Geometry: final body of the model. Coordinates: model frame, mm. Face numbers are marked on the shaded views. Round coordinates to 2 decimals unless told otherwise and drop trailing zeros. Write each loop counter-clockwise with the first axis right and the second up, starting at its lowest first coordinate (ties: lowest second). Pieces come first, ordered by that corner, then holes. Notation, with made-up numbers: M 59,62 L 81,62 A12 ccw 81,68 Z; hole C 7.25,77.5 d5. An arc over 180 degrees is marked long. Use one line per item in the form item = value. Start each with the question number.
Item 1: Section query A-A (z = 0). Return loops of the section in (x, y), and give its area (3 significant figures).
Item 2: Pull-direction query (Z, two-part tool) for the marked faces 1, 2 and 3; classes: pulls with the +Z half, pulls with the -Z half, needs draft (parallel to the pull), parting line crosses it, or undercut.
Item 3: Pin query (flat end, axial travel): pin 1 Ø3 at (x, y) = (-11.5, -2.5) entering from +Z; pin 2 Ø2 at (x, y) = (-11.5, -4.5) entering from -Z; pin 3 Ø2 at (x, y) = (-9, -5) entering from +Z; pin 4 Ø5 at (x, y) = (-3, -2.5) entering from +Z (3 decimals). Return the tip coordinate at first contact, or that it passes through.
Item 4: Ray query, probe 1 along Z at (x, y) = (-15, -9.25); probe 2 along Z at (x, y) = (-8.75, -12.25); probe 3 along X at (y, z) = (-17.5, 2). Return the intervals inside material, ascending.
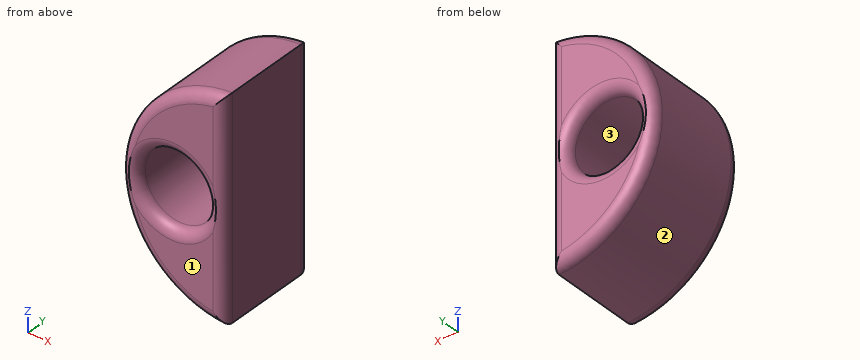
from build123d import *

# Parameters (mm, degrees)
F1_DEPTH    = 20
F2_R        = 6.5
F3_DEPTH    = 20
F4_T1_DEPTH = 49.9499687109
F4_T4_ANGLE = 202.9591024792
F4_T6_ANGLE = 202.9591024792


# Not quite as in the source:
# - a fillet or chamfer that OpenCascade refuses, or shapes differently, is made with other operations: its cross-section is extruded or revolved along the edge and cut away or added


with BuildPart() as f1:
    # F0 (on Front) → F1 (new body)
    with BuildSketch(Plane.XZ):
        with BuildLine():
            Line((-1, 0), (-1, 19.9749843554))
            ThreePointArc((-1, 19.9749843554), (-20, 0), (-1, -19.9749843554))
            Line((-1, -19.9749843554), (-1, 0))
        make_face()
    extrude(amount=F1_DEPTH)

    # F2 (on face) → F3 (cut)
    with BuildSketch(Plane.XZ.offset(20)):
        with Locations((-10.5, 0)):
            Circle(F2_R)
    extrude(amount=-F3_DEPTH, mode=Mode.SUBTRACT)

    # F4: fillet of radius 2 on 6 edges, made by hand

    # F4_s2 → F4_t1 (cut)
    with BuildSketch(Plane.XY.offset(-24.9749843554)):
        with BuildLine():
            ThreePointArc((-1, -18), (-1.5857864376, -19.4142135624), (-3, -20))
            Line((-3, -20), (-1, -20))
            Line((-1, -20), (-1, -18))
        make_face()
        with BuildLine():
            ThreePointArc((-1, -2), (-1.5857864376, -0.5857864376), (-3, 0))
            Line((-3, 0), (-1, 0))
            Line((-1, 0), (-1, -2))
        make_face()
    extrude(amount=F4_T1_DEPTH, mode=Mode.SUBTRACT)

    # F4_s3 → F4_t4 (revolve, cut)
    with BuildSketch(Plane(origin=(0, 0, 0), x_dir=(0, 1, 0), z_dir=(0.9799957963, 0, -0.1990181884))):
        with BuildLine():
            ThreePointArc((-18, 20), (-19.4142135624, 19.4142135624), (-20, 18))
            Line((-20, 18), (-20, 20))
            Line((-20, 20), (-18, 20))
        make_face()
    revolve(axis=Axis((0, -20, 0), (0, -1, 0)), revolution_arc=F4_T4_ANGLE, mode=Mode.SUBTRACT)

    # F4_s5 → F4_t6 (revolve, cut)
    with BuildSketch(Plane(origin=(0, 0, 0), x_dir=(0, 1, 0), z_dir=(0.9799957963, 0, -0.1990181884))):
        with BuildLine():
            ThreePointArc((-2, 20), (-0.5857864376, 19.4142135624), (0, 18))
            Line((0, 18), (0, 20))
            Line((0, 20), (-2, 20))
        make_face()
    revolve(axis=Axis((0, 0, 0), (0, -1, 0)), revolution_arc=F4_T6_ANGLE, mode=Mode.SUBTRACT)

    # F4_s7 → F4_t8 (revolve, cut)
    with BuildSketch(Plane.XY):
        with BuildLine():
            ThreePointArc((-2, 0), (-3.4142135624, -0.5857864376), (-4, -2))
            Line((-4, -2), (-4, 0))
            Line((-4, 0), (-2, 0))
        make_face()
    revolve(axis=Axis((-10.5, 0, 0), (0, -1, 0)), mode=Mode.SUBTRACT)

    # F4_s9 → F4_t10 (revolve, cut)
    with BuildSketch(Plane.XY):
        with BuildLine():
            ThreePointArc((-2, -20), (-3.4142135624, -19.4142135624), (-4, -18))
            Line((-4, -18), (-4, -20))
            Line((-4, -20), (-2, -20))
        make_face()
    revolve(axis=Axis((-10.5, -20, 0), (0, -1, 0)), mode=Mode.SUBTRACT)


solid = f1.part
Working result:
q1.outline = M -20,-18 A2 ccw -18.5,-19.94 A2 ccw -17,-18 L -17,-2 A2 ccw -18.5,-0.06 A2 ccw -20,-2 Z; M -4,-18 A2 ccw -2.5,-19.94 A2 ccw -1,-18 L -1,-2 A2 ccw -2.5,-0.06 A2 ccw -4,-2 Z
q1.area = 113 mm²
q2.face_1 = needs draft
q2.face_2 = parting line crosses it
q2.face_3 = undercut
q3.pin_1 = 17.32
q3.pin_2 = -17.02
q3.pin_3 = 18.33
q3.pin_4 = 19.975
q4.probe_1 = -13.23 to -4.69, 4.69 to 13.23
q4.probe_2 = -17.98 to -6.26, 6.26 to 17.98
q4.probe_3 = -19.9 to -16.68, -4.32 to -1
